The drawing under review shows one solid part. Ordinate dimensions are in mm from its lowest x, y, z. A direction names the side the tool comes from. Round coordinates to 2 decimals unless told otherwise and drop trailing zeros.
1) To check wall thickness, follow L1, parallel to Y at x = 2.45, z = 16. State the ranges of the line that lie inside material, in increasing order.
2) Mouldability with a two-part tool opening along Z and no side actions: class the marked faces 3 and 4 as pulls with the +Z half, pulls with the -Z half, needs draft (parallel to the pull), parting line crosses it, or undercut.
3) Machinability: for the marked faces 1 and 2, which of the approach directions +Z, -Z, +X, -X, +Y, -Y give a long, thin tool a straight path to every point of the face, cutting with its end or side? Answer none if there is none.
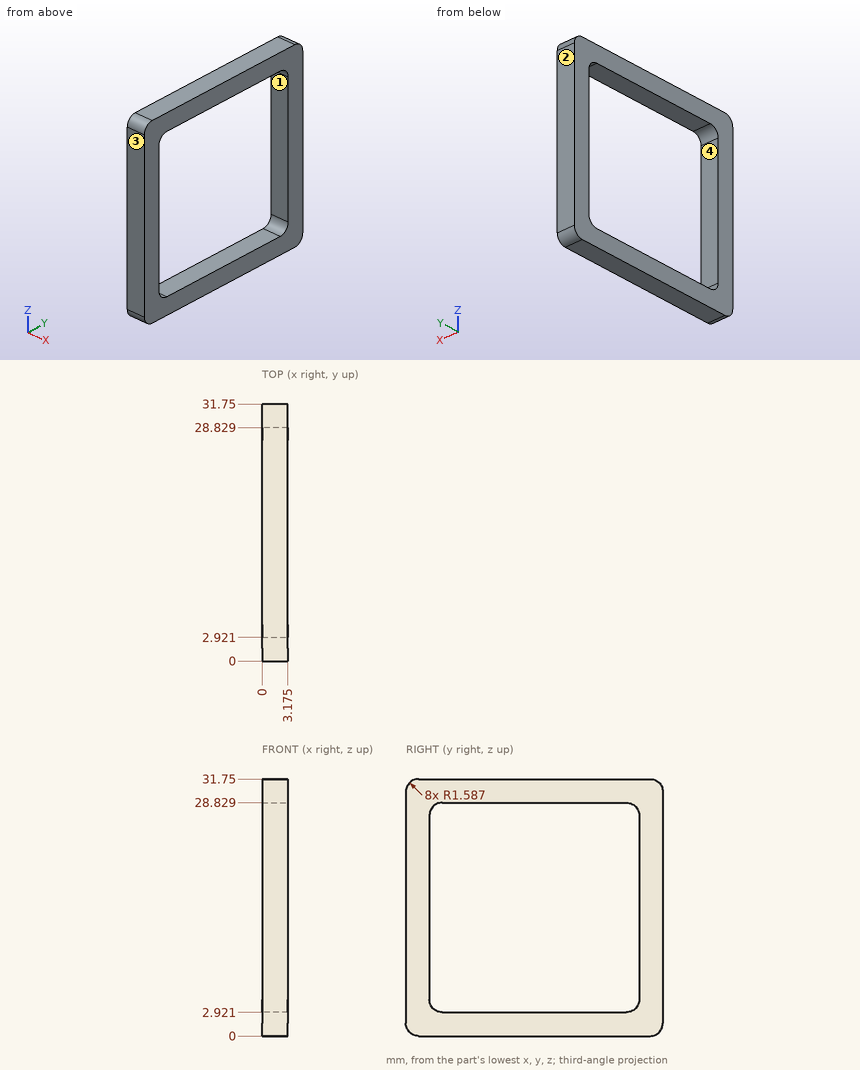
Answer below:
1. L1: y = 0 to 2.92, 28.83 to 31.75
2. face 3: needs draft
2. face 4: undercut
3. face 1: +X, -X
3. face 2: +Z, -Z, +X, -X, +Y
